Here's the drawing with two shaded views (mm, measured from the low corner). I have some questions. A direction names the side the tool comes from. Give positions to 0.01 mm unless a question says otherwise; leave off trailing zeros. Loops run counter-clockwise (first coordinate to the right, second up) from the corner with the lowest first, then second, coordinate; pieces in that order, holes last. Notation, with made-up numbers: (-32, -24) - (15, -24) arc R35 cw to (15, 12) - close; hole circle Ø11 at (47.5, 26). An arc over 180 degrees is marked (long way). Write each question's results on one line, items separated by ' | '. Start each with the question number.
1) I want a section at A-A, the plane z = 5.5. Write out the boundary of the cut face in (x, y), and give its area (3 significant figures).
2) On a 3-axis mill with a long thin cutter (end or side, diameter ignored), from which of +Z, -Z, +X, -X, +Y, -Y can I reach the whole of each face in a straight line? I mean the marked faces 1 and 2. Say none if no direction works.
3) If I drill on probe 1 along Y at (x, z) = (111, 2); probe 2 along X at (y, z) = (84, 11.5) (1 decimal); probe 3 along X at (y, z) = (77, 22), over which ranges is the centre line in solid material (lowest first)? Write a range as [from, to].
4) I want a section at B-B, the plane x = 140.5. Write out the boundary of the cut face in (y, z), and give its area (3 significant figures).
5) I'm going to push a flat-ended pin straight in: pin 1 (1 mm diameter, centred on x = 59.5, z = 22, fed in from +Y). Where does the tip first touch, or does it pass through?
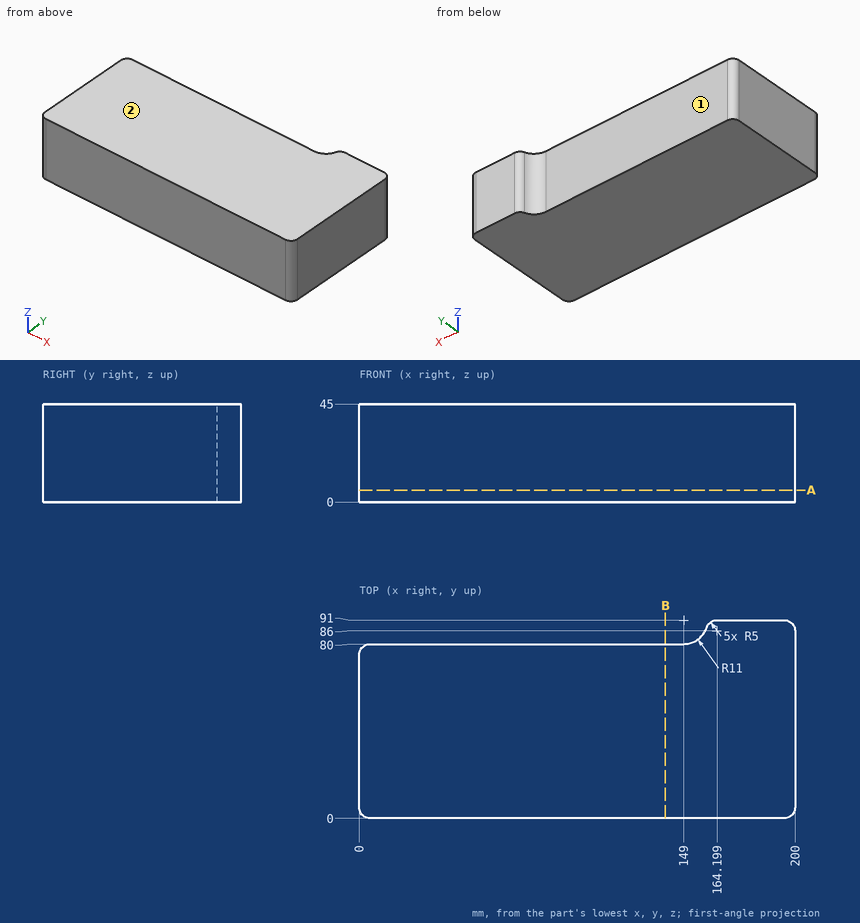
Answers:
1) outline: (0, 5) arc R5 ccw to (5, 0) - (195, 0) arc R5 ccw to (200, 5) - (200, 86) arc R5 ccw to (195, 91) - (164.2, 91) arc R5 ccw to (159.45, 87.56) arc R11 cw to (149, 80) - (5, 80) arc R5 ccw to (0, 75) - close | area: 16,400 mm2
2) face 1: +Z, -Z, -X, +Y | face 2: +Z, +X, -X, +Y, -Y
3) probe 1: y = [0, 80] | probe 2: x = [157.5, 200] | probe 3: x = [0.42, 200]
4) outline: (0, 0) - (80, 0) - (80, 45) - (0, 45) - close | area: 3,600 mm2
5) pin 1: stops at y = 80
